Geometry check sheet. Reference: the model listing, model coordinates, mm. Face numbers are marked on the shaded views. A direction names the side the tool comes from. Give positions to 0.01 mm unless a question says otherwise; leave off trailing zeros. Write each loop counter-clockwise with the first axis right and the second up, starting at its lowest first coordinate (ties: lowest second). Pieces come first, ordered by that corner, then holes. Notation, with made-up numbers: (76.5, -27.75) - (102.5, -27.75) arc R19 ccw to (102.5, -4.75) - close; hole circle Ø11 at (31, 12). An arc over 180 degrees is marked (long way). One line per question, with ' | ' between items. Start each with the question number.
Q1. Gauge pin test, flat ends, axial feed: P1, Ø4, axis at x = -70, z = 8, coming from the +Y side; P2, Ø4.5, axis at x = -67, y = -127.35, coming from the +Z side; P3, Ø5, axis at x = -73, z = 7, coming from the +Y side. Record the tip position at first contact, or that the pin passes through.
Q2. Set-up check for the marked faces 1, 2 and 3: record each of +Z, -Z, +X, -X, +Y, -Y from which the full face is reachable in a straight line by a thin tool's end or side.
Q3. Section check B-B on x = -82.5. Record the boundary of the cut face in (y, z), and give its area (3 significant figures).
Q4. Section check C-C on y = -277. Record the boundary of the cut face in (x, z).
Q5. Section check A-A on x = -89.5. Record the boundary of the cut face in (y, z), and give its area (3 significant figures).
Q6. Thickness scan on L1, parallel to X at y = -301.75, z = 6.25; L2, parallel to Z at x = -89.5, y = -299.75; L3, parallel to Z at x = -76, y = -177.5. Record the ranges inside material, lowest first. Write a range as [from, to].
```python
from build123d import *

# Parameters (mm, degrees)
SKETCH1_R           = 2
BOSS_EXTRUDE1_DEPTH = 5
SKETCH2_W           = 58
SKETCH2_H           = 10
BOSS_EXTRUDE2_DEPTH = 10
SKETCH3_R           = 3
CUT_EXTRUDE1_DEPTH  = 11


with BuildPart() as part:
    # Sketch1 → Boss-Extrude1 (new body)
    with BuildSketch(Plane.XY):
        with BuildLine():
            Line((-75.497650797, -127.154118822), (-79.5, -297.353946086))
            Line((-79.5, -297.353946086), (-96, -297.353946086))
            Line((-96, -297.353946086), (-96, -307.353946086))
            Line((-96, -307.353946086), (-38, -307.353946086))
            Line((-38, -307.353946086), (-38, -297.353946086))
            Line((-38, -297.353946086), (-54.5, -297.353946086))
            Line((-54.5, -297.353946086), (-58.502349203, -127.154118822))
            ThreePointArc((-58.502349203, -127.154118822), (-67, -118.853946086), (-75.497650797, -127.154118822))
        make_face()
        with Locations((-67, -167.353946086)):
            Circle(SKETCH1_R, mode=Mode.SUBTRACT)
        with Locations((-67, -127.353946086)):
            Circle(SKETCH1_R, mode=Mode.SUBTRACT)
    extrude(amount=BOSS_EXTRUDE1_DEPTH)

    # Sketch2 → Boss-Extrude2 (add)
    with BuildSketch(Plane.XY.offset(2.5)):
        with Locations((-67, -302.353946086)):
            Rectangle(SKETCH2_W, SKETCH2_H)
    extrude(amount=BOSS_EXTRUDE2_DEPTH)

    # Sketch3 → Cut-Extrude1 (cut, through all)
    with BuildSketch(Plane(origin=(0, -297.353946086, 0), x_dir=(1, 0, 0), z_dir=(0, 1, 0))):
        with Locations((-89.5, -6.25)):
            Circle(SKETCH3_R)
        with Locations((-44.5, -6.25)):
            Circle(SKETCH3_R)
    extrude(amount=-CUT_EXTRUDE1_DEPTH, mode=Mode.SUBTRACT)


solid = part.part
```
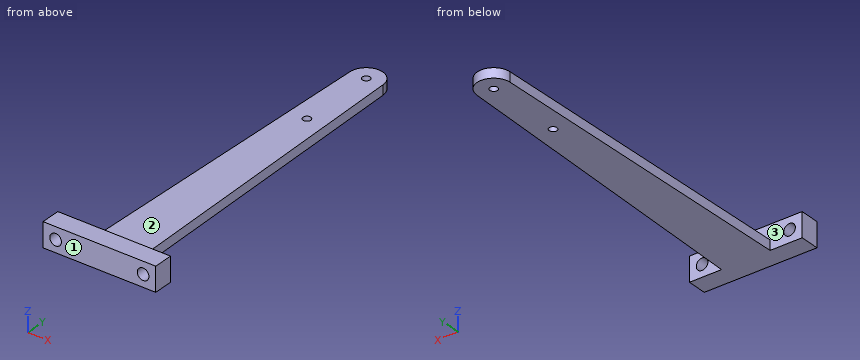
Working result:
1) P1: stops at y = -297.35 | P2: stops at z = 5 | P3: stops at y = -120.14
2) face 1: +Z, -Z, +X, -X, -Y | face 2: +Z, +X, -X, +Y | face 3: +Z, +Y
3) outline: (-307.35, 0) - (-297.35, 0) - (-297.35, 12.5) - (-307.35, 12.5) - close | area: 125 mm2
4) outline: (-79.02, 0) - (-54.98, 0) - (-54.98, 5) - (-79.02, 5) - close
5) outline: (-307.35, 0) - (-297.35, 0) - (-297.35, 3.25) - (-307.35, 3.25) - close; (-307.35, 9.25) - (-297.35, 9.25) - (-297.35, 12.5) - (-307.35, 12.5) - close | area: 65.0 mm2
6) L1: x = [-96, -92.5], [-86.5, -47.5], [-41.5, -38] | L2: z = [0, 3.25], [9.25, 12.5] | L3: z = [0, 5]
